Input: part model. Units: mm. Frame: model coordinates. A direction names the side the tool comes from. Round coordinates to 2 decimals unless told otherwise and drop trailing zeros. Loops run counter-clockwise (first coordinate to the right, second up) from the corner with the lowest first, then second, coordinate; pieces in that order, holes last. Notation, with made-up numbers: (59, 66) - (88, 66) arc R24 cw to (88, 86) - close; hole circle Ø11 at (46.5, 33). An arc over 180 degrees is marked (long way). One line per question, with ' | ' between items. Start each with the question number.
Item 1: Set-up query: faces 4 (the face through (-3, -8, -16)), 5 (the face through (4, -11, 16)), 6 (the face through (-2.38, 10.74, -14.79)). Return all of +Z, -Z, +X, -X, +Y, -Y with unobstructed straight access to the full face (end or side cutting, diameter ignored); none if empty.
Item 2: Material intervals for line 1 along Z through (x, y) = (-13.5, -3); line 2 along Z through (x, y) = (0, -15.75); line 3 along X through (y, z) = (5, 8), sorted ascending.
Item 3: Section C-C, the plane y = -13. Return loops of the section in (x, z).
Item 4: First-contact query: pin 1 (12 mm diameter, centred on x = 6, z = 31.5, fed in from -Y); pin 2 (4 mm diameter, centred on y = -3, z = 14, fed in from +X); pin 3 (1 mm diameter, centred on x = 5.5, z = 2, fed in from +Y). Flat tips, straight axial feed; report the tip coordinate or a pass-through.
Item 5: Section D-D, the plane x = -12. Return loops of the section in (y, z).
Item 6: Draft query along X for faces 1 (the face through (3, -8, -16)), 2 (the face through (0, 0, -32)), 3 (the face through (9.139, 14.334, 7.888)). Return one class per face: pulls with the +X half, pulls with the -X half, needs draft (parallel to the pull), parting line crosses it, or undercut.
Item 7: Section B-B, the plane z = 8. Return loops of the section in (x, y), plus the area to 3 significant figures.
```python
from build123d import *

# Parameters (mm, degrees)
F0_R      = 17
F1_DEPTH  = 16
F2_R      = 11
F3_DEPTH  = 32
F4_SIZE   = 2
F5_R      = 11
F6_DEPTH  = 32
F7_SIZE   = 2
F9_R      = 6
F10_DEPTH = 3.001
F11_R     = 4
F12_DEPTH = 31.001
F15_DEPTH = 12.001
F17_DEPTH = 12.001


with BuildPart() as f1:
    # F0 (on Top) → F1 (new body)
    with BuildSketch(Plane.XY):
        Circle(F0_R)
    extrude(amount=F1_DEPTH)

    # F2 (on face) → F3 (join)
    with BuildSketch(Plane(origin=(0, 0, 0), x_dir=(1, 0, 0), z_dir=(0, 0, -1))):
        Circle(F2_R)
    extrude(amount=F3_DEPTH)

    # F4
    f4_edges = [f1.edges().sort_by_distance(p)[0] for p in [
        (-11, 0, -32),
    ]]
    chamfer(f4_edges, length=F4_SIZE)

    # F5 (on face) → F6 (join)
    with BuildSketch(Plane.XY.offset(16)):
        Circle(F5_R)
    extrude(amount=F6_DEPTH)

    # F7
    f7_edges = [f1.edges().sort_by_distance(p)[0] for p in [
        (-11, 0, 48),
    ]]
    chamfer(f7_edges, length=F7_SIZE)

    # F9 (on offset) → F10 (cut, through all)
    with BuildSketch(Plane.XZ.offset(14)):
        with Locations((0, 8)):
            Circle(F9_R)
    extrude(amount=F10_DEPTH, mode=Mode.SUBTRACT)

    # F11 (on face) → F12 (cut, through all)
    with BuildSketch(Plane.XZ.offset(14)):
        with Locations((0, 8)):
            Circle(F11_R)
    extrude(amount=-F12_DEPTH, mode=Mode.SUBTRACT)

    # F14 (on offset) → F15 (cut, through all)
    with BuildSketch(Plane.XZ.offset(5)):
        with BuildLine():
            ThreePointArc((-3, 26), (0, 23), (3, 26))
            Line((3, 26), (3, 38))
            ThreePointArc((3, 38), (0, 41), (-3, 38))
            Line((-3, 38), (-3, 26))
        make_face()
    extrude(amount=F15_DEPTH, mode=Mode.SUBTRACT)

    # F16 (on offset) → F17 (cut, through all)
    with BuildSketch(Plane.XZ.offset(5)):
        with BuildLine():
            Line((3, -22), (3, -10))
            ThreePointArc((3, -10), (0, -7), (-3, -10))
            Line((-3, -10), (-3, -22))
            ThreePointArc((-3, -22), (0, -25), (3, -22))
        make_face()
    extrude(amount=F17_DEPTH, mode=Mode.SUBTRACT)


solid = f1.part
```
Return value:
1) face 4: -Y | face 5: +Z | face 6: -Z
2) line 1: 0 to 16 | line 2: 0 to 2, 14 to 16 | line 3: -16.25 to -4, 4 to 16.25
3) outline: (-10.95, 0) - (10.95, 0) - (10.95, 16) - (-10.95, 16) - close; hole circle Ø8 at (0, 8)
4) pin 1: y = -10.58 | pin 2: x = 16.97 | pin 3: y = 16.25
5) outline: (-12.04, 0) - (12.04, 0) - (12.04, 16) - (-12.04, 16) - close
6) face 1: undercut | face 2: needs draft | face 3: parting line crosses it
7) outline: (-6, -15.91) - (-6, -14) - (-4, -14) - (-4, 16.52) arc R17 ccw to start; (4, -14) - (6, -14) - (6, -15.91) arc R17 ccw to (4, 16.52) - close | area: 630 mm2
